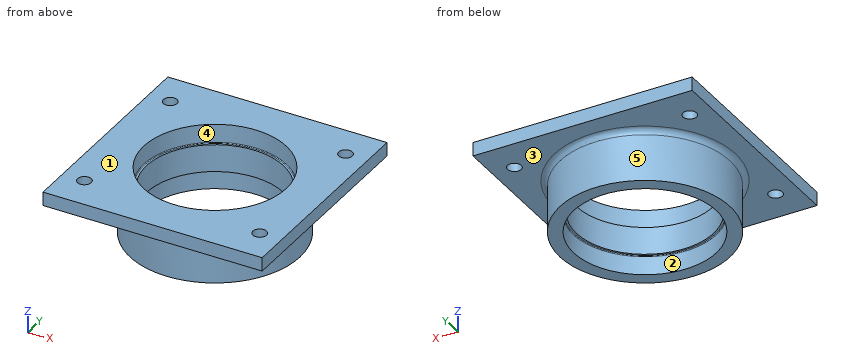
```python
from build123d import *

# Parameters (mm, degrees)
SKETCH1_R             = 31
SKETCH1_R_2           = 26
BOSS_EXTRUDE1_DEPTH   = 7
SKETCH2_R             = 31
SKETCH2_R_2           = 25
BOSS_EXTRUDE3_DEPTH   = 10
SKETCH3_R             = 31
SKETCH3_R_2           = 26
BOSS_EXTRUDE4_DEPTH   = 7
FILLET1_R             = 0.3
SKETCH4_W             = 80
SKETCH4_H             = 80
SKETCH4_R             = 31
BOSS_EXTRUDE5_DEPTH   = 5
FILLET2_R             = 2
M6X1_0_TAPPED_HOLE1_D = 5


with BuildPart() as part:
    # Sketch1 → Boss-Extrude1 (new body)
    with BuildSketch(Plane.XY):
        Circle(SKETCH1_R)
        Circle(SKETCH1_R_2, mode=Mode.SUBTRACT)
    extrude(amount=BOSS_EXTRUDE1_DEPTH)

    # Sketch2 → Boss-Extrude3 (add)
    with BuildSketch(Plane.XY.offset(7)):
        Circle(SKETCH2_R)
        Circle(SKETCH2_R_2, mode=Mode.SUBTRACT)
    extrude(amount=BOSS_EXTRUDE3_DEPTH)

    # Sketch3 → Boss-Extrude4 (add)
    with BuildSketch(Plane.XY.offset(17)):
        Circle(SKETCH3_R)
        Circle(SKETCH3_R_2, mode=Mode.SUBTRACT)
    extrude(amount=BOSS_EXTRUDE4_DEPTH)

    # Fillet1
    fillet1_edges = [part.edges().sort_by_distance(p)[0] for p in [
        (-26, 0, 7),
        (-26, 0, 17),
    ]]
    fillet(fillet1_edges, radius=FILLET1_R)

    # Sketch4 → Boss-Extrude5 (add)
    with BuildSketch(Plane.XY.offset(24)):
        Rectangle(SKETCH4_W, SKETCH4_H)
        Circle(SKETCH4_R, mode=Mode.SUBTRACT)
    extrude(amount=-BOSS_EXTRUDE5_DEPTH)

    # Fillet2
    fillet2_edges = [part.edges().sort_by_distance(p)[0] for p in [
        (-31, 0, 19),
    ]]
    fillet(fillet2_edges, radius=FILLET2_R)

    # M6x1.0 Tapped Hole1 (through all)
    with Locations(Plane.XY.offset(24)):
        with Locations((-32, 27.5), (32, 27.5), (32, -27.5), (-32, -27.5)):
            Hole(M6X1_0_TAPPED_HOLE1_D / 2)


solid = part.part
```
For this review, take the finished solid that the model builds, in its own axes (mm). Face numbers are marked on the shaded views. A direction names the side the tool comes from. Coordinates: 2 decimals unless noted, no trailing zeros. Loops run counter-clockwise (first coordinate to the right, second up) from the corner with the lowest first, then second, coordinate; pieces in that order, holes last. Notation, with made-up numbers: (78.5, 15) - (128.5, 15) arc R33 ccw to (128.5, 45) - close; hole circle Ø4 at (-20.5, 38.5). An arc over 180 degrees is marked (long way). Use one line per item in the form item = value. Start each with the question number.
1) For the marked faces 1 and 2, list the 3-axis set-ups (+Z, -Z, +X, -X, +Y, -Y) from which the entire face can be reached by the end or side of a thin tool; tool diameter is ignored.
2) Draft analysis for pull direction X (two halves, no side actions). For the marked faces 3, 4 and 5, state which applies: released by +X, released by -X, zero draft, split by the parting line, or undercut.
3) Take a section at C-C (z = 2.25). State the section outline as (x, y) points.
4) To check wall thickness, follow probe 1 along Y at (x, z) = (32, 21.35); probe 2 along Y at (x, z) = (0, 19.75); probe 3 along Y at (x, z) = (1, 8.25). State the ranges of each line that lie inside material, in increasing order. Write a range as from..to.
5) Take a section at D-D (x = 32). State how many separate pieces and enclosed holes the cut face has, plus the area to 3 significant figures.
6) Take a section at A-A (y = 0). State the section outline as (x, z) points, plus the area to 3 significant figures.
7) For pin 1 (1.5 mm diameter, centred on x = 6.5, z = 7.5, fed in from +Y); pin 2 (10 mm diameter, centred on y = -0.5, z = 9.5, fed in from +X); pin 3 (1 mm diameter, centred on y = -20.5, z = 7, fed in from +X); pin 4 (4 mm diameter, centred on y = 20, z = 18, fed in from -X), all flat-tipped, find the tip position at first contact; note any pin that passes through.
From the geometry:
q1.face_1 = +Z, +X, -X, +Y, -Y
q1.face_2 = -Z
q2.face_3 = zero draft
q2.face_4 = undercut
q2.face_5 = split by the parting line
q3.outline = circle Ø62 at (0, 0); hole circle Ø52 at (0, 0)
q4.probe_1 = -40..-30, -25..25, 30..40
q4.probe_2 = -40..-26, 26..40
q4.probe_3 = -30.98..-24.98, 24.98..30.98
q5.separate_pieces = 3
q5.enclosed_holes = 0
q5.area = 352 mm2
q6.outline = (-40, 19) - (-33, 19) arc R2 cw to (-31, 17) - (-31, 0) - (-26, 0) - (-26, 6.7) arc R0.3 cw to (-25.7, 7) - (-25, 7) - (-25, 17) - (-25.7, 17) arc R0.3 cw to (-26, 17.3) - (-26, 24) - (-40, 24) - close; (25, 7) - (25.7, 7) arc R0.3 cw to (26, 6.7) - (26, 0) - (31, 0) - (31, 17) arc R2 cw to (33, 19) - (40, 19) - (40, 24) - (26, 24) - (26, 17.3) arc R0.3 cw to (25.7, 17) - (25, 17) - close
q6.area = 352 mm2
q7.pin_1 = 30.46
q7.pin_2 = 31
q7.pin_3 = 23.69
q7.pin_4 = -40
